```python
from build123d import *

# Parameters (mm, degrees)
F1_DEPTH = 92.71
F4_DEPTH = 539.242


with BuildPart() as f1:
    # F0 (on Top) → F1 (new body)
    with BuildSketch(Plane.XY):
        Polygon((22.950954, -39.752218), (22.950954, 39.752218), (-45.901908, 0), align=None)
    extrude(amount=F1_DEPTH)

    # F3 (on offset) → F4 (cut)
    with BuildSketch(Plane.XZ.offset(254)):
        Polygon((-61.28243, 96.673079), (-61.28243, 0), (-28.304175, 0), (-28.304175, 40.58408), (8.569154, 40.58408), (-30.900886, 92.518345), (-33.757269, 96.673079), align=None)
    extrude(amount=-F4_DEPTH, mode=Mode.SUBTRACT)


solid = f1.part
```
CAD build for the part. Positions are in the model's coordinates, mm. A direction names the side the tool comes from. Round coordinates to 2 decimals unless told otherwise and drop trailing zeros. Order: outer loops, then holes, each group sorted by start corner. A loop starts at its lowest first (then second) coordinate and runs counter-clockwise, first axis right, second up. Notation, with made-up numbers: (-14.5, 32.5) -> (26.5, 32.5) arc R21 ccw to (26.5, 48.5) -> close; hole circle Ø5 at (54, 76). An arc over 180 degrees is marked (long way). Write item = value, one per line.
(1) Cut at D-D (x = -24.5). Write the cut outline in (y, z).
Answers follow:
outline = (-12.36, 0) -> (12.36, 0) -> (12.36, 40.58) -> (-12.36, 40.58) -> close; (-12.36, 84.1) -> (12.36, 84.1) -> (12.36, 92.71) -> (-12.36, 92.71) -> close
(2) Flat gauge pins, fed straight in: P1, Ø2, axis at x = -22.5, z = 24.5, coming from the -Y side; P2, Ø2, axis at x = -16.5, z = 26.5, coming from the +Y side; P3, Ø2, axis at x = 13.5, z = 61.5, coming from the +Y side; P4, Ø3, axis at x = -15.5, y = 5.5, coming from the -Z side. Where does each tip first touch, or does it go through?
Answers follow:
P1 = -14.09
P2 = 17.55
P3 = 34.87
P4 = 0
(3) Drill centre lines: L1, parallel to Z at x = 6, y = 26.5; L2, parallel to Z at x = -26, y = -3.5; L3, parallel to X at y = -6, z = 40.5. Where is each one in solid material? Low to high.
Answers follow:
L1 = 0 to 40.58, 43.96 to 92.71
L2 = 0 to 40.58, 86.07 to 92.71
L3 = -28.3 to 22.95
(4) 3-axis set-ups, long thin cutter, end or side, ignore diameter. For faces 4 (the flat face through (-28.304, 0, 20)), 5 (the flat face through (-6, 0, 40.584)), 6 (the flat face through (2.335, 27.85, 35.405)): which of +Z, -Z, +X, -X, +Y, -Y reach the whole face in a straight line?
Answers follow:
face_4 = -Z, -X, +Y, -Y
face_5 = -X, +Y, -Y
face_6 = +Z, -Z, -X, +Y
(5) Cut at B-B (x = -5.5). Write the cut outline in (y, z), plus the area to 3 significant figures.
Answers follow:
outline = (-23.33, 0) -> (23.33, 0) -> (23.33, 40.58) -> (-23.33, 40.58) -> close; (-23.33, 59.1) -> (23.33, 59.1) -> (23.33, 92.71) -> (-23.33, 92.71) -> close
area = 3,460 mm²
(6) Pull direction Z, two halves, no side cores. Call faces 1 (the flat face through (2, 1, 92.71)), 2 (the flat face through (-6.504, -0.44, 60.417)), 3 (the flat face through (7.58, -30.88, 45.71)): +Z half, -Z half, draft (parallel to the pull), parting line (faces both ways), or undercut.
Answers follow:
face_1 = +Z half
face_2 = undercut
face_3 = draft
(7) Cut at A-A (y = 4.5). Write the cut outline in (x, z).
Answers follow:
outline = (-31.03, 92.71) -> (-30.9, 92.52) -> (8.57, 40.58) -> (-28.3, 40.58) -> (-28.3, 0) -> (22.95, 0) -> (22.95, 92.71) -> close
(8) Cut at C-C (z = 8). Write the cut outline in (x, y).
Answers follow:
outline = (-28.3, -10.16) -> (22.95, -39.75) -> (22.95, 39.75) -> (-28.3, 10.16) -> close
